Verification items for the finished model (mm, model axes). Face numbers are marked on the shaded views. A direction names the side the tool comes from. Round coordinates to 2 decimals unless told otherwise and drop trailing zeros. Write each loop counter-clockwise with the first axis right and the second up, starting at its lowest first coordinate (ties: lowest second). Pieces come first, ordered by that corner, then holes. Notation, with made-up numbers: (57.5, -28) - (97.5, -28) arc R19 cw to (97.5, 0) - close; hole circle Ø3 at (28, -15.75). An arc over 180 degrees is marked (long way). Answer as a JSON object with one key per item and string values.
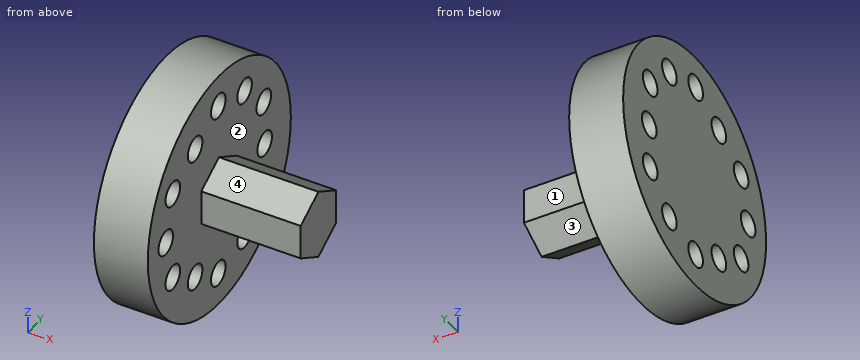
```python
from build123d import *

# Parameters (mm, degrees)
SKETCH1_R           = 24.5
SKETCH1_R_2         = 2.5
BOSS_EXTRUDE1_DEPTH = 10.85
BOSS_EXTRUDE2_DEPTH = 20


with BuildPart() as part:
    # Sketch1 → Boss-Extrude1 (new body)
    with BuildSketch(Plane(origin=(0, 0, 0), x_dir=(0, 0, -1), z_dir=(1, 0, 0))):
        Circle(SKETCH1_R)
        with Locations((0, 15.545215773)):
            Circle(SKETCH1_R_2, mode=Mode.SUBTRACT)
        with Locations((13.612452271, -8.304784227)):
            Circle(SKETCH1_R_2, mode=Mode.SUBTRACT)
        with Locations((-13.927155569, -8.304784227)):
            Circle(SKETCH1_R_2, mode=Mode.SUBTRACT)
        with Locations((8.842648351, 15.233673041)):
            Circle(SKETCH1_R_2, mode=Mode.SUBTRACT)
        with Locations((15.431105619, 8.645215773)):
            Circle(SKETCH1_R_2, mode=Mode.SUBTRACT)
        with Locations((17.842648351, -0.354784227)):
            Circle(SKETCH1_R_2, mode=Mode.SUBTRACT)
        with Locations((8.842648351, -15.943241495)):
            Circle(SKETCH1_R_2, mode=Mode.SUBTRACT)
        with Locations((-0.157351649, -18.354784227)):
            Circle(SKETCH1_R_2, mode=Mode.SUBTRACT)
        with Locations((-9.157351649, -15.943241495)):
            Circle(SKETCH1_R_2, mode=Mode.SUBTRACT)
        with Locations((-18.157351649, -0.354784227)):
            Circle(SKETCH1_R_2, mode=Mode.SUBTRACT)
        with Locations((-15.745808917, 8.645215773)):
            Circle(SKETCH1_R_2, mode=Mode.SUBTRACT)
        with Locations((-9.157351649, 15.233673041)):
            Circle(SKETCH1_R_2, mode=Mode.SUBTRACT)
    extrude(amount=BOSS_EXTRUDE1_DEPTH)

    # Sketch4 → Boss-Extrude2 (add)
    with BuildSketch(Plane(origin=(10.85, 0, 0), x_dir=(0, 0, -1), z_dir=(1, 0, 0))):
        Polygon((7, -0.130869058), (3.5, 5.931308769), (-3.5, 5.931308769), (-7, -0.130869058), (-3.5, -6.193046884), (3.5, -6.193046884), align=None)
    extrude(amount=BOSS_EXTRUDE2_DEPTH)


solid = part.part
```
1. Cross-section at D-D (y = -1). Record the boundary of the cut face in (x, z).
Completed:
{"outline": "(0, -24.48) - (10.85, -24.48) - (10.85, -20.26) - (0, -20.26) - close; (0, -15.43) - (10.85, -15.43) - (10.85, -6.5) - (30.85, -6.5) - (30.85, 6.5) - (10.85, 6.5) - (10.85, 15.74) - (0, 15.74) - close; (0, 20.57) - (10.85, 20.57) - (10.85, 24.48) - (0, 24.48) - close"}
2. Material ranges on probe 1 along Y at (x, z) = (5.5, -14.5); probe 2 along Y at (x, z) = (3.5, -9); probe 3 along X at (y, z) = (-4.5, -14.5), recorded low to high. Write a range as from..to.
Completed:
{"probe 1": "y = -19.75..-10.64, -5.97..6.33, 10.97..19.75", "probe 2": "y = -22.79..-18.44, -13.45..12.74, 17.73..22.79", "probe 3": "x = 0..10.85"}
3. Cross-section at A-A (x = 25). Record the boundary of the cut face in (y, z), plus the area to 3 significant figures.
Completed:
{"outline": "(-6.19, -3.5) - (-0.13, -7) - (5.93, -3.5) - (5.93, 3.5) - (-0.13, 7) - (-6.19, 3.5) - close", "area": "127 mm^2"}
4. Access from +Z, -Z, +X, -X, +Y, -Y to the whole of each face (thin tool, end or side, straight path). Record for the marked faces 1, 2, 3 and 4.
Completed:
{"face 1": "+Z, -Z, +X, +Y", "face 2": "+X", "face 3": "-Z, +X, +Y", "face 4": "+Z, +X, -Y"}
5. Cross-section at B-B (z = -10). Record the boundary of the cut face in (x, y).
Completed:
{"outline": "(0, -22.37) - (10.85, -22.37) - (10.85, -18.16) - (0, -18.16) - close; (0, -13.73) - (10.85, -13.73) - (10.85, 13.02) - (0, 13.02) - close; (0, 17.45) - (10.85, 17.45) - (10.85, 22.37) - (0, 22.37) - close"}
6. Cross-section at C-C (x = 2). Count the separate pieces of the cut face and the enclosed holes in it, plus the area to 3 significant figures.
Completed:
{"separate pieces": "1", "enclosed holes": "12", "area": "1,650 mm^2"}
7. Go/stop test with flat-tipped pins: pin 1 (4 mm diameter, centred on y = -15.94, z = 9.16, fed in from -X); pin 2 (10 mm diameter, centred on x = 23.5, y = -4.5, fed in from +Z); pin 3 (7.5 mm diameter, centred on x = 22, z = 0.5, fed in from -Y); pin 4 (6 mm diameter, centred on x = 9, y = -17, fed in from -Z). Record where each tip stops, or that it passes through.
Completed:
{"pin 1": "passes through", "pin 2": "stops at z = 7", "pin 3": "stops at y = -6.19", "pin 4": "stops at z = -20.11"}
